Can you work these out from the drawing? Everything is in mm from the part's minimum corner. Coordinates: 2 decimals unless noted, no trailing zeros. Loops run counter-clockwise (first coordinate to the right, second up) from the corner with the lowest first, then second, coordinate; pieces in that order, holes last. Notation, with made-up numbers: (-7, 48.5) -> (30, 48.5) arc R27 ccw to (30, 82.5) -> close; hole circle Ø6 at (76.25, 46.5). An arc over 180 degrees is marked (long way). One line per question, with ' | ' between items.
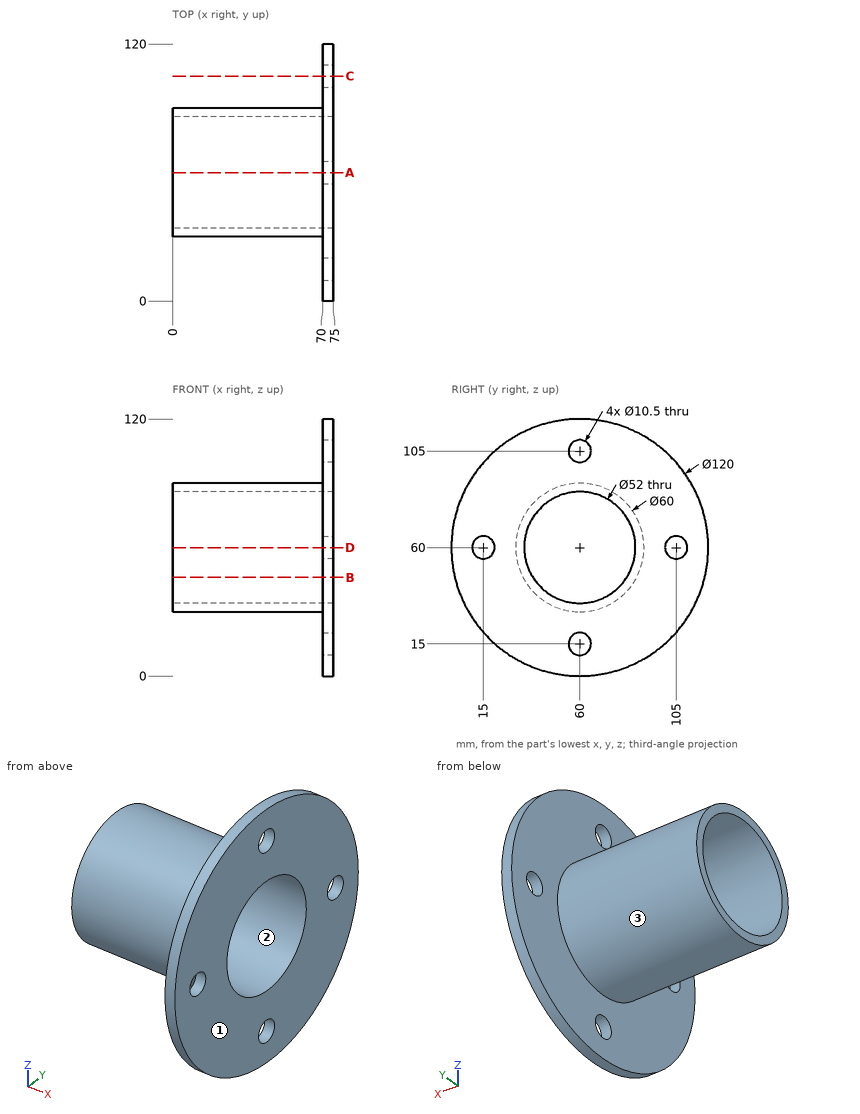
Q1. Please list where these lines run through material, in increasing order: L1, parallel to Y at x = 72.9, z = 60; L2, parallel to Z at x = 32, y = 61; L3, parallel to X at y = 105.5, z = 47. Write a range as [from, to].
Values follow:
L1: y = [0, 9.75], [20.25, 34], [86, 99.75], [110.25, 120] | L2: z = [30.02, 34.02], [85.98, 89.98] | L3: x = [70, 75]
Q2. Imagine slicing it at B-B on z = 46. Write out the boundary of the cut face in (x, y).
Values follow:
outline: (0, 33.47) -> (70, 33.47) -> (70, 1.66) -> (75, 1.66) -> (75, 38.09) -> (0, 38.09) -> close; (0, 81.91) -> (75, 81.91) -> (75, 118.34) -> (70, 118.34) -> (70, 86.53) -> (0, 86.53) -> close
Q3. For pin 1 (17 mm diameter, centred on y = 60, z = 15, fed in from -X); pin 2 (1 mm diameter, centred on x = 58.5, y = 82, fed in from -Z); pin 3 (4 mm diameter, centred on x = 23.5, y = 64.5, fed in from +Z); pin 4 (12 mm diameter, centred on y = 60, z = 105, fed in from +X), each with a flat end and sliding along its axis, tell me the tip position at first contact or that it passes through.
Values follow:
pin 1: stops at x = 70 | pin 2: stops at z = 39.08 | pin 3: stops at z = 89.9 | pin 4: stops at x = 75
Q4. Imagine slicing it at C-C on y = 105. Write out the boundary of the cut face in (x, z).
Values follow:
outline: (70, 20.31) -> (75, 20.31) -> (75, 54.75) -> (70, 54.75) -> close; (70, 65.25) -> (75, 65.25) -> (75, 99.69) -> (70, 99.69) -> close
Q5. Imagine slicing it at A-A on y = 60. Write out the boundary of the cut face in (x, z), plus the area to 3 significant figures.
Values follow:
outline: (0, 30) -> (70, 30) -> (70, 20.25) -> (75, 20.25) -> (75, 34) -> (0, 34) -> close; (0, 86) -> (75, 86) -> (75, 99.75) -> (70, 99.75) -> (70, 90) -> (0, 90) -> close; (70, 0) -> (75, 0) -> (75, 9.75) -> (70, 9.75) -> close; (70, 110.25) -> (75, 110.25) -> (75, 120) -> (70, 120) -> close | area: 795 mm2
Q6. We'd pull the mould along Z, two halves only. Please class the marked faces 1, 2 and 3: released by +Z, released by -Z, zero draft, split by the parting line, or undercut.
Values follow:
face 1: zero draft | face 2: undercut | face 3: split by the parting line
